```python
from build123d import *

# Parameters (mm, degrees)
SKETCH_1_W          = 91
SKETCH_1_H          = 48
EXTRUDE_1_DEPTH     = 4
SKETCH_2_W          = 75
SKETCH_2_H          = 28
CUT_EXTRUDE_1_DEPTH = 52.596996037
FILLET_2_R          = 8
SKETCH_3_R          = 1.65
CUT_EXTRUDE_2_DEPTH = 52.596996037
SKETCH_5_W          = 13
SKETCH_5_H          = 20
EXTRUDE_2_DEPTH     = 4
SKETCH_6_W          = 13
SKETCH_6_H          = 5
EXTRUDE_3_DEPTH     = 30
EXTRUDE_4_DEPTH     = 13
SKETCH_8_R          = 2.5
CUT_EXTRUDE_3_DEPTH = 30
CUT_EXTRUDE_4_DEPTH = 107.644268482
FILLET_3_R          = 0.5
FILLET_4_R          = 4


with BuildPart() as part:
    # 草图1 → 凸台-拉伸1 (new body)
    with BuildSketch(Plane.XY):
        Rectangle(SKETCH_1_W, SKETCH_1_H)
    extrude(amount=EXTRUDE_1_DEPTH)

    # 草图2 → 切除-拉伸1 (cut, through all)
    with BuildSketch(Plane.XY.offset(4)):
        Rectangle(SKETCH_2_W, SKETCH_2_H)
    extrude(amount=-CUT_EXTRUDE_1_DEPTH, mode=Mode.SUBTRACT)

    # 圆角2
    fillet_2_edges = [part.edges().sort_by_distance(p)[0] for p in [
        (37.5, 14, 2),
        (37.5, -14, 2),
        (-37.5, -14, 2),
        (-37.5, 14, 2),
    ]]
    fillet(fillet_2_edges, radius=FILLET_2_R)

    # 草图3 → 切除-拉伸2 (cut, through all)
    with BuildSketch(Plane.XY.offset(4)):
        with Locations((-41.5, 20)):
            Circle(SKETCH_3_R)
        with Locations((-41.5, -20)):
            Circle(SKETCH_3_R)
        with Locations((41.5, 20)):
            Circle(SKETCH_3_R)
        with Locations((41.5, -20)):
            Circle(SKETCH_3_R)
    extrude(amount=-CUT_EXTRUDE_2_DEPTH, mode=Mode.SUBTRACT)

    # 草图5 → 凸台-拉伸2 (add)
    with BuildSketch(Plane(origin=(0, 0, 0), x_dir=(-1, 0, 0), z_dir=(0, 0, -1))):
        with Locations((-39, -34)):
            Rectangle(SKETCH_5_W, SKETCH_5_H)
        with Locations((39, -34)):
            Rectangle(SKETCH_5_W, SKETCH_5_H)
    extrude(amount=-EXTRUDE_2_DEPTH)

    # 草图6 → 凸台-拉伸3 (add)
    with BuildSketch(Plane.XY.offset(4)):
        with Locations((-39, -41.5)):
            Rectangle(SKETCH_6_W, SKETCH_6_H)
        with Locations((39, -41.5)):
            Rectangle(SKETCH_6_W, SKETCH_6_H)
    extrude(amount=EXTRUDE_3_DEPTH)

    # 草图7 → 凸台-拉伸4 (add)
    with BuildSketch(Plane(origin=(45.5, 0, 0), x_dir=(0, 0, -1), z_dir=(1, 0, 0))):
        Polygon((-4, -27), (-14, -39), (-4, -39), align=None)
    extrude_4 = extrude(amount=-EXTRUDE_4_DEPTH)

    # 镜向2: 凸台-拉伸4 across plane
    add(extrude_4.mirror(Plane(origin=(0, 0, 0), x_dir=(0, 0, 1), z_dir=(1, 0, 0))))

    # 草图8 → 切除-拉伸3 (cut)
    with BuildSketch(Plane.XZ.offset(44)):
        with Locations((39, 29)):
            Circle(SKETCH_8_R)
        with Locations((-39, 29)):
            Circle(SKETCH_8_R)
        with Locations((39, 14)):
            Circle(SKETCH_8_R)
        with Locations((-39, 14)):
            Circle(SKETCH_8_R)
    extrude(amount=-CUT_EXTRUDE_3_DEPTH, mode=Mode.SUBTRACT)

    # 草图9 → 切除-拉伸4 (cut, through all)
    with BuildSketch(Plane.ZY.offset(45.5)):
        Polygon((9, -33), (9, -39), (14, -39), align=None)
    extrude(amount=-CUT_EXTRUDE_4_DEPTH, mode=Mode.SUBTRACT)

    # 圆角3
    fillet_3_edges = [part.edges().sort_by_distance(p)[0] for p in [
        (39, -39, 9),
        (39, -33, 9),
        (-39, -33, 9),
        (-39, -39, 9),
    ]]
    fillet(fillet_3_edges, radius=FILLET_3_R)

    # 圆角4
    fillet_4_edges = [part.edges().sort_by_distance(p)[0] for p in [
        (-45.5, 24, 2),
        (45.5, 24, 2),
    ]]
    fillet(fillet_4_edges, radius=FILLET_4_R)


solid = part.part
```
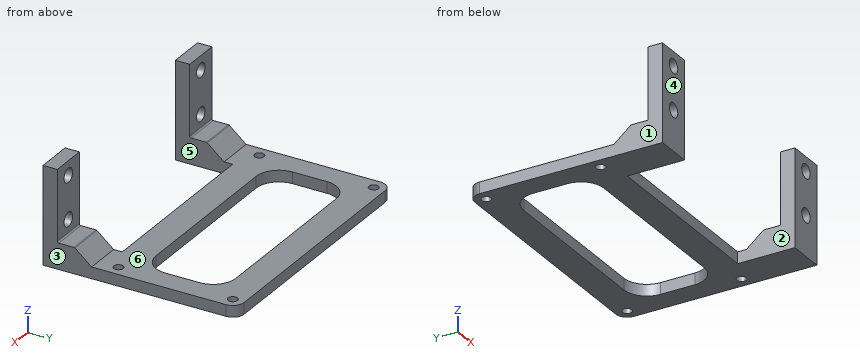
Model file for the job. Use its own axes, mm. Face numbers are marked on the shaded views. A direction names the side the tool comes from. Coordinates: 2 decimals unless noted, no trailing zeros. Order: outer loops, then holes, each group sorted by start corner. A loop starts at its lowest first (then second) coordinate and runs counter-clockwise, first axis right, second up. Notation, with made-up numbers: (-14, -32.75) -> (44, -32.75) arc R30 ccw to (44, 3.25) -> close; hole circle Ø3 at (47.5, -39). An arc over 180 degrees is marked (long way). Answer as a JSON object with one key per item and string values. Group by question number.
1) Cut at D-D, the plane y = -20. Write the cut outline in (x, z), then the cut area to 3 significant figures.
2) Cut at B-B, the plane x = 1. Write the cut outline in (y, z), then the cut area to 3 significant figures.
3) Cut at A-A, the plane z = 7. Write the cut outline in (x, y).
4) Pull direction X, two halves, no side cores. Call the marked faces 1, 2 and 3: +X half, -X half, draft (parallel to the pull), parting line (faces both ways), or undercut.
5) Drill centre lines: L1, parallel to Y at x = -41.5, z = 2.75; L2, parallel to Z at x = 39, y = -41; L3, parallel to Y at x = 35, z = 21. Where is each one in solid material? Low to high.
6) Which spindle directions (+Z, -Z, +X, -X, +Y, -Y) get a long thin tool onto all of the face, cutting with end or side? Do the marked faces 4, 5 and 6. Say none if no direction does.
7) Cut at C-C, the plane z = 14. Write the cut outline in (x, y).
8) Flat gauge pins, fed straight in: pin 1 (4.5 mm diameter, centred on x = 6, z = 1, fed in from -Y); pin 2 (6.5 mm diameter, centred on x = -39, z = 14, fed in from -Y); pin 3 (6 mm diameter, centred on x = 40.5, y = -35, fed in from +Z); pin 4 (15.5 mm diameter, centred on x = -22.5, y = 10, fed in from +Z). Where does each tip first touch, or does it go through?
Check values:
{
 "1": {"outline": "(-45.5, 0) -> (-43.15, 0) -> (-43.15, 4) -> (-45.5, 4) -> close; (-39.85, 0) -> (39.85, 0) -> (39.85, 4) -> (-39.85, 4) -> close; (43.15, 0) -> (45.5, 0) -> (45.5, 4) -> (43.15, 4) -> close", "area": "338 mm²"},
 "2": {"outline": "(-24, 0) -> (-14, 0) -> (-14, 4) -> (-24, 4) -> close; (14, 0) -> (24, 0) -> (24, 4) -> (14, 4) -> close", "area": "80.0 mm²"},
 "3": {"outline": "(-45.5, -44) -> (-32.5, -44) -> (-32.5, -30.6) -> (-45.5, -30.6) -> close; (32.5, -44) -> (45.5, -44) -> (45.5, -30.6) -> (32.5, -30.6) -> close"},
 "4": {"face 1": "-X half", "face 2": "undercut", "face 3": "+X half"},
 "5": {"L1": "y = -44 to -21.65, -18.35 to 18.35, 21.65 to 24", "L2": "z = 0 to 11.5, 16.5 to 26.5, 31.5 to 34", "L3": "y = -44 to -39"},
 "6": {"face 4": "+Z, -Z, +X, -X, -Y", "face 5": "+Z, -Z, -Y", "face 6": "+Z, +X, -X, +Y"},
 "7": {"outline": "(-45.5, -44) -> (-41.5, -44) -> (-41.5, -39) -> (-45.5, -39) -> close; (-36.5, -44) -> (-32.5, -44) -> (-32.5, -39) -> (-36.5, -39) -> close; (32.5, -44) -> (36.5, -44) -> (36.5, -39) -> (32.5, -39) -> close; (41.5, -44) -> (45.5, -44) -> (45.5, -39) -> (41.5, -39) -> close"},
 "8": {"pin 1": "stops at y = -24", "pin 2": "stops at y = -44", "pin 3": "stops at z = 9", "pin 4": "stops at z = 4"}
}
